from build123d import *

# Parameters (mm, degrees)
SKETCH_1_W      = 6.2
SKETCH_1_H      = 6.2
EXTRUDE_1_DEPTH = 3.5
SKETCH_2_R      = 1.75
EXTRUDE_2_DEPTH = 0.9
SKETCH_3_W      = 0.3
SKETCH_3_H      = 0.8
EXTRUDE_3_DEPTH = 14.35


with BuildPart() as part:
    # Эскиз1 → Бобышка-Вытянуть1 (new body)
    with BuildSketch(Plane(origin=(0, 0, 0), x_dir=(1, 0, 0), z_dir=(0, 1, 0))):
        Rectangle(SKETCH_1_W, SKETCH_1_H)
    extrude(amount=EXTRUDE_1_DEPTH)

    # Эскиз2 → Бобышка-Вытянуть2 (add)
    with BuildSketch(Plane(origin=(0, 3.5, 0), x_dir=(1, 0, 0), z_dir=(0, 1, 0))):
        with Locations(Location((0, 0, 0), (0, 0, 90))):
            Circle(SKETCH_2_R)
    extrude(amount=EXTRUDE_2_DEPTH)

    # Эскиз3 → Бобышка-Вытянуть3 (add)
    with BuildSketch(Plane.XZ):
        with Locations((0, 2.5)):
            Rectangle(SKETCH_3_W, SKETCH_3_H)
        with Locations((0, -2.5)):
            Rectangle(SKETCH_3_W, SKETCH_3_H)
    extrude(amount=EXTRUDE_3_DEPTH)


solid = part.part
CAD build for the part. Positions are in the model's coordinates, mm. A direction names the side the tool comes from. Round coordinates to 2 decimals unless told otherwise and drop trailing zeros. Loops run counter-clockwise (first coordinate to the right, second up) from the corner with the lowest first, then second, coordinate; pieces in that order, holes last. Notation, with made-up numbers: (74.25, 4.25) - (93.25, 4.25) arc R22 cw to (93.25, 26.25) - close; hole circle Ø5 at (5.25, 53.25). An arc over 180 degrees is marked (long way). Put each result on its own line as item: value.
1. Slice it at C-C on z = 0. List the corners of the cut face in (x, y), and give its area (4 significant figures).
Geometry check:
outline: (-3.1, 0) - (3.1, 0) - (3.1, 3.5) - (1.75, 3.5) - (1.75, 4.4) - (-1.75, 4.4) - (-1.75, 3.5) - (-3.1, 3.5) - close
area: 24.85 mm²
2. 3-axis set-ups, long thin cutter, end or side, ignore diameter. For faces 1 (the flat face through (-1.4, 3.5, 1.3)), 2 (the flat face through (3.1, 2, 0)): which of +Z, -Z, +X, -X, +Y, -Y reach the whole face in a straight line?
Geometry check:
face 1: +Y
face 2: +Z, -Z, +X, +Y, -Y
3. Slice it at D-D on x = 2.75. List the corners of the cut face in (y, z), and give its area (3 significant figures).
Geometry check:
outline: (0, -3.1) - (3.5, -3.1) - (3.5, 3.1) - (0, 3.1) - close
area: 21.7 mm²
4. Pin check, flat tips, straight feed: P1, Ø3, axis at x = 1.5, y = -8, coming from the +Z side; P2, Ø0.6, axis at y = -9.5, z = 2.5, coming from the +X side; P3, Ø1.9, axis at x = 1, z = 0.5, coming from the -Y side. Stop position of each tip, or through.
Geometry check:
P1: z = 2.9
P2: x = 0.15
P3: y = 0
5. Wall check: line 1 (Z direction, x = 0, y = -11); line 2 (Y direction, x = 2, z = 0.75); line 3 (Y direction, x = -0.25, z = 0.75). Give the ranges that are in metal, low to high.
Geometry check:
line 1: -2.9 to -2.1, 2.1 to 2.9
line 2: 0 to 3.5
line 3: 0 to 4.4
6. Slice it at B-B on x = -0.5. List the corners of the cut face in (y, z).
Geometry check:
outline: (0, -3.1) - (3.5, -3.1) - (3.5, -1.68) - (4.4, -1.68) - (4.4, 1.68) - (3.5, 1.68) - (3.5, 3.1) - (0, 3.1) - close
7. Slice it at A-A on y = -8.75. List the corners of the cut face in (x, z).
Geometry check:
outline: (-0.15, -2.9) - (0.15, -2.9) - (0.15, -2.1) - (-0.15, -2.1) - close; (-0.15, 2.1) - (0.15, 2.1) - (0.15, 2.9) - (-0.15, 2.9) - close
